For this review, use the dimensioned drawing (mm, ordinates from the lowest corner) and the shaded views. A direction names the side the tool comes from. Round coordinates to 2 decimals unless told otherwise and drop trailing zeros. Order: outer loops, then holes, each group sorted by start corner. A loop starts at its lowest first (then second) coordinate and runs counter-clockwise, first axis right, second up. Notation, with made-up numbers: (43.5, 44) - (90.5, 44) arc R23 cw to (90.5, 63) - close; hole circle Ø11 at (24, 26). An arc over 180 degrees is marked (long way). Write item = value, one per line.
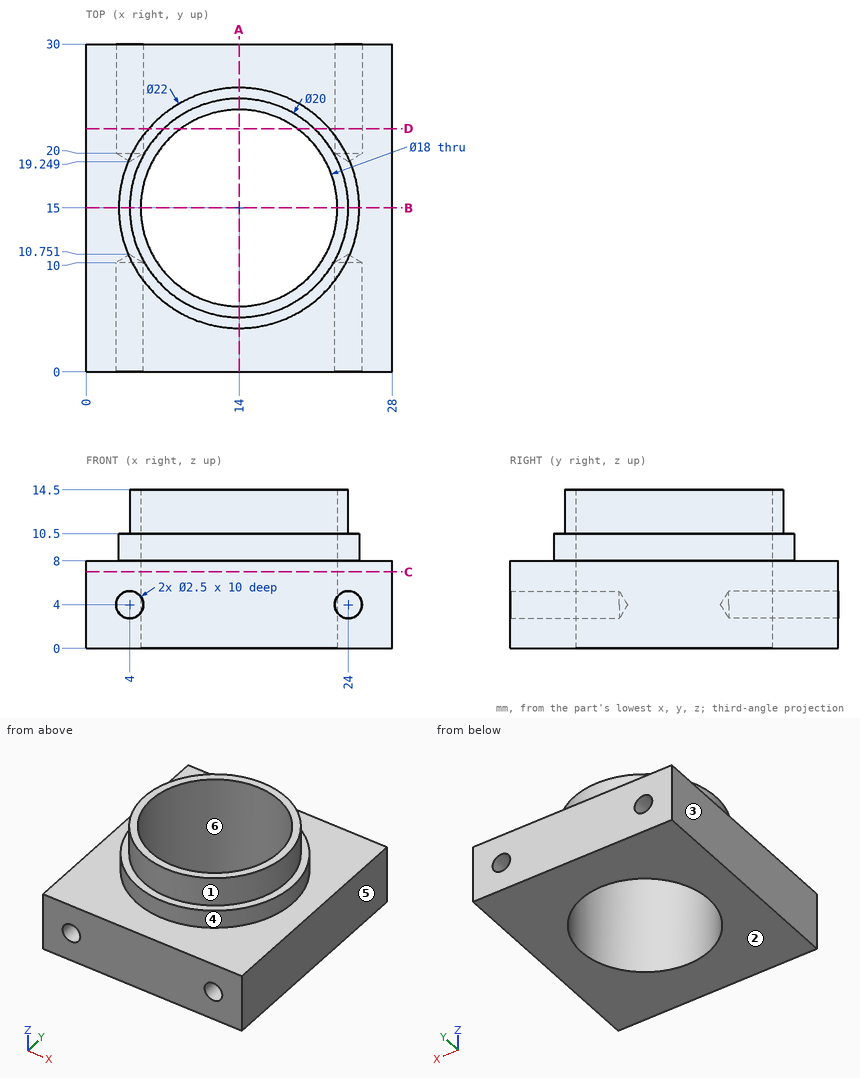
Item 1: Take a section at C-C, the plane z = 7. State the section outline as (x, y) points, and give its area (3 significant figures).
Data:
outline = (0, 0) - (28, 0) - (28, 30) - (0, 30) - close; hole circle Ø18 at (14, 15)
area = 586 mm2
Item 2: Take a section at D-D, the plane y = 22.25. State the section outline as (x, z) points.
Data:
outline = (0, 0) - (8.67, 0) - (8.67, 14.5) - (7.11, 14.5) - (7.11, 10.5) - (5.73, 10.5) - (5.73, 8) - (0, 8) - close; (19.33, 0) - (28, 0) - (28, 8) - (22.27, 8) - (22.27, 10.5) - (20.89, 10.5) - (20.89, 14.5) - (19.33, 14.5) - close; hole circle Ø2.5 at (4, 4); hole circle Ø2.5 at (24, 4)
Item 3: For line 1 along X through (y, z) = (3.5, 4); line 2 along Z through (x, y) = (4, 27); line 3 along Z through (x, y) = (24.75, 27), list the stretches that pass through material, from the lowest coordinate up. Write a range as [from, to].
Data:
line_1 = [0, 2.75], [5.25, 22.75], [25.25, 28]
line_2 = [0, 2.75], [5.25, 8]
line_3 = [0, 3], [5, 8]
Item 4: For the marked faces 1 and 2, list the 3-axis set-ups (+Z, -Z, +X, -X, +Y, -Y) from which the entire face can be reached by the end or side of a thin tool; tool diameter is ignored.
Data:
face_1 = +Z
face_2 = -Z, +X, -X, +Y, -Y
Item 5: Take a section at B-B, the plane y = 15. State the section outline as (x, z) points, and give its area (3 significant figures).
Data:
outline = (0, 0) - (5, 0) - (5, 14.5) - (4, 14.5) - (4, 10.5) - (3, 10.5) - (3, 8) - (0, 8) - close; (23, 0) - (28, 0) - (28, 8) - (25, 8) - (25, 10.5) - (24, 10.5) - (24, 14.5) - (23, 14.5) - close
area = 98.0 mm2
Item 6: The part is to be moulded in two halves that separate along X. For the marked faces 3, 4, 5 and 6, say which applies: +X half, -X half, draft (parallel to the pull), parting line (faces both ways), or undercut.
Data:
face_3 = -X half
face_4 = parting line
face_5 = +X half
face_6 = undercut
Item 7: Insertion check: P1, Ø3, axis at x = 24, z = 4, coming from the -Y side; P2, Ø2, axis at x = 4, z = 4, coming from the +Y side; P3, Ø5, axis at x = 17, z = 12.5, coming from the +Y side; P4, Ø2, axis at x = 24, z = 4, coming from the -Y side. Each pin has a flat end and moves straight along its axis. Give the tip position at first contact, or say it passes through.
Data:
P1 = 0
P2 = 19.85
P3 = 25.9
P4 = 10.15
Item 8: Take a section at A-A, the plane x = 14. State the section outline as (y, z) points, and give its area (3 significant figures).
Data:
outline = (0, 0) - (6, 0) - (6, 14.5) - (5, 14.5) - (5, 10.5) - (4, 10.5) - (4, 8) - (0, 8) - close; (24, 0) - (30, 0) - (30, 8) - (26, 8) - (26, 10.5) - (25, 10.5) - (25, 14.5) - (24, 14.5) - close
area = 114 mm2
